For this review, take the finished solid that the model builds, in its own axes (mm). Coordinates: 2 decimals unless noted, no trailing zeros. Write item = value, one per line. Start each with the question number.
1) Wall thickness on probe 1 along X at (y, z) = (83, 0.15); probe 2 along X at (y, z) = (56, 0.5); probe 3 along Y at (x, z) = (316.23, 0.8): over which ranges is each line inside the solid? List them lowest first. Write a range as [from, to].
2) Insertion check: pin 1 Ø21.5 at (x, y) = (316.23, 334.04) entering from -Z. The pin has a flat end and moves straight along its axis. Give the tip position at first contact, or say it passes through.
3) Consider section A-A on z = 1.6. State how many separate pieces and enclosed holes the cut face has, and give its area (3 significant figures).
from build123d import *

# Parameters (mm, degrees)
F0_W     = 558.8
F0_H     = 457.2
F0_R     = 5.588
F0_R_2   = 6.74624
F0_R_3   = 41.275
F1_DEPTH = 2.778125


with BuildPart() as f1:
    # F0 (on Top) → F1 (new body)
    with BuildSketch(Plane.XY):
        with Locations((279.4, 228.6)):
            Rectangle(F0_W, F0_H)
        with Locations((22.352, 22.352)):
            Circle(F0_R, mode=Mode.SUBTRACT)
        with BuildLine():
            ThreePointArc((43.18, 113.157), (46.899744, 122.137256), (55.88, 125.857))
            Line((55.88, 125.857), (119.38, 125.857))
            ThreePointArc((119.38, 125.857), (128.360256, 122.137256), (132.08, 113.157))
            Line((132.08, 113.157), (132.08, 56.007))
            ThreePointArc((132.08, 56.007), (128.360256, 47.026744), (119.38, 43.307))
            Line((119.38, 43.307), (55.88, 43.307))
            ThreePointArc((55.88, 43.307), (46.899744, 47.026744), (43.18, 56.007))
            Line((43.18, 56.007), (43.18, 113.157))
        make_face(mode=Mode.SUBTRACT)
        with Locations((55.88, 202.057)):
            Circle(F0_R_2, mode=Mode.SUBTRACT)
        with Locations((240.03, 202.057)):
            Circle(F0_R_2, mode=Mode.SUBTRACT)
        with Locations((279.4, 84.582)):
            Circle(F0_R_3, mode=Mode.SUBTRACT)
        with Locations((536.702, 22.352)):
            Circle(F0_R, mode=Mode.SUBTRACT)
        with BuildLine():
            Line((439.42, 125.857), (502.92, 125.857))
            ThreePointArc((502.92, 125.857), (511.900256, 122.137256), (515.62, 113.157))
            Line((515.62, 113.157), (515.62, 56.007))
            ThreePointArc((515.62, 56.007), (511.900256, 47.026744), (502.92, 43.307))
            Line((502.92, 43.307), (439.42, 43.307))
            ThreePointArc((439.42, 43.307), (430.439744, 47.026744), (426.72, 56.007))
            Line((426.72, 56.007), (426.72, 113.157))
            ThreePointArc((426.72, 113.157), (430.439744, 122.137256), (439.42, 125.857))
        make_face(mode=Mode.SUBTRACT)
        with Locations((424.18, 202.057)):
            Circle(F0_R_2, mode=Mode.SUBTRACT)
        with Locations((132.08, 334.039272)):
            Circle(F0_R_2, mode=Mode.SUBTRACT)
        with Locations((22.352, 434.848)):
            Circle(F0_R, mode=Mode.SUBTRACT)
        with Locations((316.23, 334.039272)):
            Circle(F0_R_2, mode=Mode.SUBTRACT)
        with Locations((500.38, 334.039272)):
            Circle(F0_R_2, mode=Mode.SUBTRACT)
        with Locations((536.702, 434.848)):
            Circle(F0_R, mode=Mode.SUBTRACT)
    extrude(amount=F1_DEPTH)


solid = f1.part
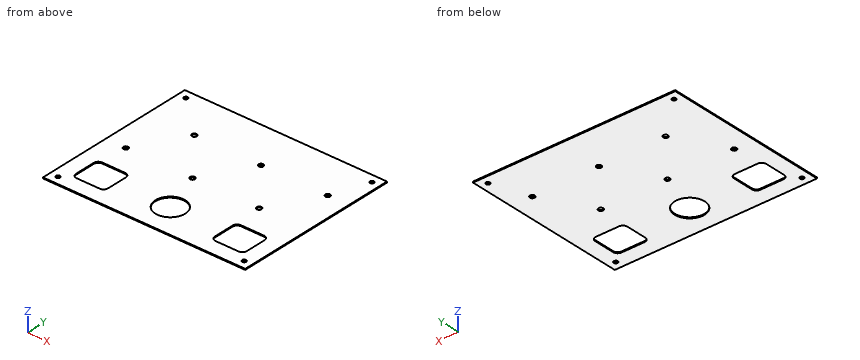
Answer sheet:
q1.probe_1 = [0, 43.18], [132.08, 238.16], [320.64, 426.72], [515.62, 558.8]
q1.probe_2 = [0, 43.18], [132.08, 249.62], [309.18, 426.72], [515.62, 558.8]
q1.probe_3 = [0, 65.95], [103.21, 327.29], [340.79, 457.2]
q2.pin_1 = 0
q3.separate_pieces = 1
q3.enclosed_holes = 13
q3.area = 234,000 mm2
